Autodesk Inventor part; units mm, degrees
ref_plane "YZ Plane" through (0, 0, 0) normal (1, 0, 0) x (0, 1, 0)
ref_plane "XZ Plane" through (0, 0, 0) normal (0, 1, 0) x (-1, 0, 0)
ref_plane "XY Plane" through (0, 0, 0) normal (0, 0, 1) x (1, 0, 0)
sketch "Sketch1" plane through (0, 0, 0) normal (0, 0, 1) x (1, 0, 0)
  point P0 (0, 0)
ref_plane "Work Plane1" through (0, 125.1054, -82.3097) normal (0, 0, 1) x (1, 0, 0)
sketch "Sketch2" plane through (0, 125.1054, -82.3097) normal (0, 0, 1) x (1, 0, 0)
  circle A0 centre (0.3907, 0.2373) radius 6
  circle A1 centre (0.3907, -124.7627) radius 6
  line L0 (6.3907, 6.2373) -> (-5.6093, 6.2373)
  line L1 (-5.6093, 6.2373) -> (-5.6093, -130.7627)
  line L2 (-5.6093, -130.7627) -> (6.3907, -130.7627)
  line L3 (6.3907, -130.7627) -> (6.3907, 6.2373)
  point P0 (0, -125.1054)
extrude "Extrusion1" add sketch "Sketch2" along normal blind 3
sketch "Sketch5" plane through (6.3907, -5.6573, -82.3097) normal (1, 0, 0) x (0, 0, -1)
  line L0 (0, 0) -> (0, 137)
  line L1 (0, 137) -> (-3, 137)
  line L2 (-3, 0) -> (-3, 137)
  line L3 (0, 0) -> (-3, 0)
  line L4 (-3, 0) -> (-3, 137) construction
  line L5 (-3, 68.5) -> (0, 68.5) construction
  line L6 (0, 0) -> (0, 137) construction
  line L7 (-3, 48.5) -> (0, 48.5)
  line L8 (0, 48.5) -> (0, 88.5)
  line L9 (0, 88.5) -> (-3, 88.5)
  line L10 (-3, 88.5) -> (-3, 48.5)
  line L11 (-3, 48.5) -> (0, 88.5) construction
  line L12 (0, 48.5) -> (-3, 88.5) construction
  point P0 (-82.3097, 5.6573)
  point P1 (-1.5, 68.5)
  point P2 (0, 88.5)
  point P3 (-3, 88.5)
  point P4 (-3, 48.5)
  point P5 (0, 48.5)
  dimension "d9" = 3
  dimension "d10" = 40
extrude "Extrusion4" add sketch "Sketch5" along normal blind 30 contours L7 L2 L9 L0
sketch "Sketch6" plane through (0, 125.1054, -82.3097) normal (0, 0, -1) x (-1, 0, 0)
  point P0 (0, -125.1054)
sketch "Sketch7" plane through (0, 125.1054, -79.3097) normal (0, 0, 1) x (1, 0, 0)
  line L0 (6.3907, 6.2373) -> (-5.6093, 6.2373) construction
  line L1 (-5.6093, 6.2373) -> (-5.6093, -130.7627) construction
  line L2 (-5.6093, -130.7627) -> (6.3907, -130.7627) construction
  line L3 (6.3907, -130.7627) -> (6.3907, -82.2627) construction
  line L4 (6.3907, -82.2627) -> (36.3907, -82.2627) construction
  line L5 (36.3907, -42.2627) -> (36.3907, -82.2627) construction
  line L6 (6.3907, -42.2627) -> (36.3907, -42.2627) construction
  line L7 (6.3907, -42.2627) -> (6.3907, 6.2373) construction
  line L8 (6.3907, -130.7627) -> (6.3907, -82.2627) construction
  line L9 (6.3907, -42.2627) -> (6.3907, -82.2627) construction
  circle A0 centre (15.3907, -62.2627) radius 6
  point P0 (0, -125.1054)
  point P1 (6.3907, -62.2627)
  dimension "d13" = 12
  dimension "d14" = 9
extrude "Extrusion5" cut sketch "Sketch7" against normal blind 30
properties part number "Linear rod connecting plate"
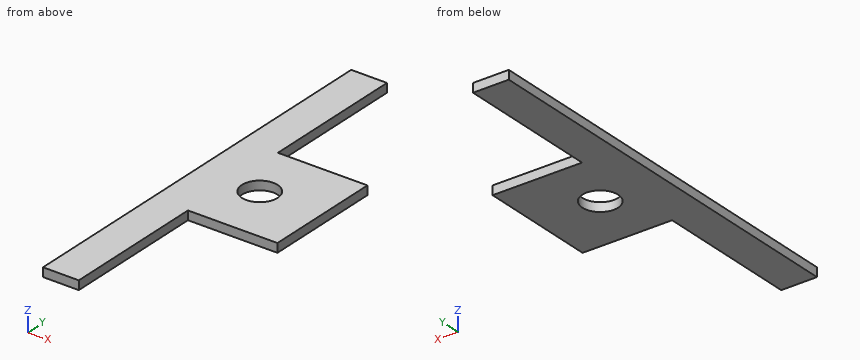
Source: CAD feature listing. Evaluate the final solid. Frame: model axes, mm. Give positions to 0.01 mm unless a question says otherwise; leave off trailing zeros. Write each loop counter-clockwise with the first axis right and the second up, starting at its lowest first coordinate (ties: lowest second). Pieces come first, ordered by that corner, then holes. Notation, with made-up numbers: (7, 45) - (13, 45) arc R29 ccw to (13, 76) - close; hole circle Ø8 at (-27, 30). An arc over 180 degrees is marked (long way). One line per item, written item: value. Start each with the question number.
Q1. Section query C-C, the plane y = 14.5. Return the cut outline in (x, z).
Q2. Section query B-B, the plane z = -81.25. Return the cut outline in (x, y), then the cut area to 3 significant figures.
Q3. Section query A-A, the plane x = 14. Return the cut outline in (y, z).
Q4. Section query D-D, the plane x = 25. Return the cut outline in (y, z), then the cut area to 3 significant figures.
Q5. Material intervals for probe 1 along X at (y, z) = (13, -80.8); probe 2 along Y at (x, z) = (14, -79.35); probe 3 along Y at (x, z) = (7.5, -80.35), sorted ascending. Write a range as from..to.
Q6. First-contact query: pin 1 Ø1.5 at (x, z) = (10, -80) entering from -Y. Flat tip, straight axial feed; report the tip coordinate or a pass-through.
Answer:
1. outline: (-5.61, -82.31) - (6.39, -82.31) - (6.39, -79.31) - (-5.61, -79.31) - close
2. outline: (-5.61, -5.66) - (6.39, -5.66) - (6.39, 42.84) - (36.39, 42.84) - (36.39, 82.84) - (6.39, 82.84) - (6.39, 131.34) - (-5.61, 131.34) - close; hole circle Ø12 at (15.39, 62.84)
2. area: 2,730 mm2
3. outline: (42.84, -82.31) - (57.01, -82.31) - (57.01, -79.31) - (42.84, -79.31) - close; (68.68, -82.31) - (82.84, -82.31) - (82.84, -79.31) - (68.68, -79.31) - close
4. outline: (42.84, -82.31) - (82.84, -82.31) - (82.84, -79.31) - (42.84, -79.31) - close
4. area: 120 mm2
5. probe 1: x = -5.61..6.39
5. probe 2: y = 42.84..57.01, 68.68..82.84
5. probe 3: y = 42.84..82.84
6. pin 1: stops at y = 42.84
